Could you check a few things on this model? Use its own coordinates, in mm. A direction names the side the tool comes from. Give positions to 0.01 mm unless a question says otherwise; leave off trailing zeros. Loops run counter-clockwise (first coordinate to the right, second up) from the corner with the lowest first, then second, coordinate; pieces in that order, holes last. Notation, with made-up numbers: M -37,38.25 L -16,38.25 A10 cw -16,53.25 Z; hole C -25,87 d10. An arc over 180 degrees is marked long. Answer in a Markdown table with one row per item. Add a question column.
Autodesk Inventor part; units mm, degrees
ref_plane "YZ Plane" through (0, 0, 0) normal (1, 0, 0) x (0, 1, 0)
ref_plane "XZ Plane" through (0, 0, 0) normal (0, 1, 0) x (-1, 0, 0)
ref_plane "XY Plane" through (0, 0, 0) normal (0, 0, 1) x (1, 0, 0)
sketch "Sketch1" plane through (0, 0, 0) normal (0, 1, 0) x (-1, 0, 0)
  line L0 (0, 0) -> (-22.8, 0)
  line L1 (-22.8, 0) -> (-22.8, -17.8)
  line L2 (-22.8, -17.8) -> (0, -17.8)
  line L3 (0, -17.8) -> (0, 0)
  dimension "d0" = 22.8
  dimension "d1" = 17.8
extrude "Extrusion1" add sketch "Sketch1" along normal blind 0.9
sketch "Sketch2" plane through (0, 0.9, 0) normal (0, 1, 0) x (1, 0, 0)
  line L0 (14.1431, 3.2431) -> (8.4863, 8.9)
  line L1 (8.4863, 8.9) -> (14.1431, 14.5569)
  line L2 (14.1431, 14.5569) -> (19.8, 8.9)
  line L3 (19.8, 8.9) -> (14.1431, 3.2431)
  line L4 (22.8, 0) -> (22.8, 17.8)
  point P0 (0, 0)
  point P1 (22.8, 8.9)
  dimension "d4" = 135
  dimension "d5" = 8
  dimension "d6" = 3
extrude "Extrusion2" add sketch "Sketch2" along normal blind 1
sketch "Sketch3" plane through (0, 0.9, 0) normal (0, 1, 0) x (1, 0, 0)
  line L0 (6, 4.4) -> (-1.5, 4.4)
  line L1 (-1.5, 4.4) -> (-1.5, 13.4)
  line L2 (-1.5, 13.4) -> (6, 13.4)
  line L3 (6, 13.4) -> (6, 4.4)
  line L4 (0, 17.8) -> (0, 0)
  point P0 (-1.5, 8.9)
  point P1 (0, 8.9)
  dimension "d9" = 7.5
  dimension "d10" = 1.5
  dimension "d11" = 9
extrude "Extrusion3" add sketch "Sketch3" along normal blind 3.2
fillet "Fillet1" radius 1.6 4 edges at (2.25, 4.1, -4.4) (2.25, 4.1, -13.4) (-0.75, 0.9, -4.4) (-0.75, 0.9, -13.4)
properties part number "rp2040"
Item 1: Suppose I cut it at B-B (y = 1.45). List the corners of the cut face in (x, z) for me.
Item 2: If we mould it in two halves opening along X, with no side actions, what happens to faces 1 (the face through (11.354, 1.393, -6.032)), 2 (the face through (16.9, 1.4, -11.8)), 3 (the face through (11.2, 0.4, 0))? For each: +X half, -X half, draft (parallel to the pull), parting line (faces both ways), or undercut.
Item 3: Suppose I cut it at C-C (z = -14). List the corners of the cut face in (x, y) for me.
Item 4: Suppose I cut it at A-A (x = 15.75). List the corners of the cut face in (y, z) for me, then the cut area to 3 significant figures.
Item 5: For P1, Ø1, axis at x = 19.5, z = -15.5, coming from the +Y side; P2, Ø5.5, axis at x = 16.5, z = -11.5, coming from the +Y side; P3, Ø1.5, axis at x = 8, y = 3, coming from the -Z side; P4, Ø1, axis at y = 2, z = -8, coming from the +X side, each with a flat end and sliding along its axis, tell me the tip position at first contact or that it passes through.
Item 6: I need wall thicknesses on L1, parallel to X at y = 1.7, z = -6.25; L2, parallel to X at y = 0.6, z = -3; L3, parallel to Y at x = 21.25, z = -8. Which ranges of each line are inside material? Lowest first, please.
Item 7: For faces 4 (the face through (6, 2, -9)), 5 (the face through (-0.74, 1.356, -12.919)), 6 (the face through (11.275, 1.393, -11.689)), which set-ups out of +Z, -Z, +X, -X, +Y, -Y let a thin tool reach every point of the face, with its end or its side?
Item 8: Suppose I cut it at D-D (y = 0.3). List the corners of the cut face in (x, z) for me.
Values found:
| question | item | result |
|---|---|---|
| 1 | outline | M -1.5,-13.01 L 0,-13.01 L 0,-13.4 L 6,-13.4 L 6,-4.4 L 0,-4.4 L 0,-4.79 L -1.5,-4.79 Z; M 8.49,-8.9 L 14.14,-14.56 L 19.8,-8.9 L 14.14,-3.24 Z |
| 2 | face 1 | undercut |
| 2 | face 2 | +X half |
| 2 | face 3 | draft |
| 3 | outline | M 0,0 L 22.8,0 L 22.8,0.9 L 14.7,0.9 L 14.7,1.9 L 13.59,1.9 L 13.59,0.9 L 0,0.9 Z |
| 4 | outline | M 0,-17.8 L 0.9,-17.8 L 0.9,-12.95 L 1.9,-12.95 L 1.9,-4.85 L 0.9,-4.85 L 0.9,0 L 0,0 Z |
| 4 | area | 24.1 mm² |
| 5 | P1 | y = 0.9 |
| 5 | P2 | y = 1.9 |
| 5 | P3 | through |
| 5 | P4 | x = 19.39 |
| 6 | L1 | -1.5 to 6, 11.14 to 17.15 |
| 6 | L2 | 0 to 22.8 |
| 6 | L3 | 0 to 0.9 |
| 7 | face 4 | +Z, -Z, +Y |
| 7 | face 5 | -Z, -X, -Y |
| 7 | face 6 | -Z, +Y |
| 8 | outline | M 0,-17.8 L 22.8,-17.8 L 22.8,0 L 0,0 Z |
